Input: part model. Units: mm. Frame: model coordinates. A direction names the side the tool comes from. Round coordinates to 2 decimals unless told otherwise and drop trailing zeros. Loops run counter-clockwise (first coordinate to the right, second up) from the corner with the lowest first, then second, coordinate; pieces in that order, holes last. Notation, with made-up numbers: (26.5, 56.25) -> (37.5, 56.25) arc R19 ccw to (37.5, 67.25) -> close; hole circle Ø2 at (2, -22). An arc over 180 degrees is marked (long way). Answer in a Markdown table with one row per item. Add a question column.
Q1. Mould query, pull axis X, two halves, no side actions, for faces 1 (the face through (-6, -15, -6)), 2 (the face through (0.1, -4.4, 8.9)), 3 (the face through (-8.49, 3.69, -8.42)). Classes: pulls with the +X half, pulls with the -X half, needs draft (parallel to the pull), parting line crosses it, or undercut.
Q2. Section A-A, the plane y = 5. Output: boundary loops of the cut face in (x, z).
Q3. Section B-B, the plane y = -4. Output: boundary loops of the cut face in (x, z), and give its area (3 significant figures).
Q4. Reachability of faces 4 (the face through (-9, -11, -3.1)), 5 (the face through (6, -15, 6)), 6 (the face through (-6, -1, 6)), 7 (the face through (-3.8, -2.25, 0.04)) from +Z, -Z, +X, -X, +Y, -Y: full face, straight path, thin tool, end or side. Return the list, or none.
Q5. Pin query (flat end, axial travel): pin 1 (6 mm diameter, centred on y = 6, z = -5.5, fed in from +X); pin 2 (7.5 mm diameter, centred on y = -11, z = -10, fed in from -X); pin 3 (1.5 mm diameter, centred on x = -6.5, z = 5, fed in from +Y); pin 4 (3 mm diameter, centred on y = -10, z = -0.5, fed in from +X). Return the tip coordinate at first contact, or that it passes through.
Q6. Section C-C, the plane y = 9.5. Output: boundary loops of the cut face in (x, z), and give its area (3 significant figures).
Q7. Ray query, L1, parallel to Z at x = 7.5, y = -6.5; L2, parallel to Z at x = -6, y = 10; L3, parallel to X at y = -3.5, z = -3.25. Return the intervals inside material, ascending. Write a range as from..to.
Autodesk Inventor part; units mm, degrees
ref_plane "Work Plane2" through (0, 0, 0) normal (0.7071, 0, -0.7071) x (0, 1, 0)
ref_plane "XZ Plane" through (0, 0, 0) normal (0, 1, 0) x (-1, 0, 0)
sketch "Sketch1" plane through (0, 0, 0) normal (0, 1, 0) x (-1, 0, 0)
  circle A0 centre (0, 0) radius 12.5
  dimension "d0" = 25
extrude "Extrusion1" add sketch "Sketch1" along normal blind 19 and the other way blind 15
sketch "Sketch2" plane through (0, 0, 0) normal (0, 0, 1) x (1, 0, 0)
  line L0 (-5.25, -15) -> (-5.25, -7.5)
  arc A0 (5.25, -7.5) -> (-5.25, -7.5) centre (0, -7.5) ccw
  line L1 (5.25, -7.5) -> (5.25, -15)
  line L2 (5.25, -15) -> (-5.25, -15)
  line L3 (-3.1, -15) -> (-3.1, -7.5)
  arc A1 (3.1, -7.5) -> (-3.1, -7.5) centre (0, -7.5) ccw
  line L4 (3.1, -7.5) -> (3.1, -15)
  line L5 (0, 0) -> (0, -15) construction
  line L6 (-12.5, -15) -> (12.5, -15)
  point P0 (0, -7.5)
  dimension "d5" = 10.5
  dimension "d6" = 6.2
extrude "Extrusion2" cut sketch "Sketch2" along normal mid plane 10.5
extrude "Extrusion3" cut sketch "Sketch2" against normal through all both and the other way through all contours L3 A1 L4 L2
pattern_circular "Circular Pattern1" count 2 over 90 about axis through (0, -10, 0) along (0, 1, 0) of "Extrusion2", "Extrusion3"
ref_plane "Work Plane2" through (0, 0, 0) normal (0.7071, 0, -0.7071) x (0, 1, 0)
sketch "Sketch5" plane through (0, 0, 0) normal (0.7071, 0, -0.7071) x (0, 1, 0)
  line L0 (19, -21.9203) -> (-2.0622, -21.9203)
  line L1 (-21.8122, 0) -> (25.8729, 0)
  line L2 (19, -12.5) -> (19, 12.5)
  line L3 (19, -21.9203) -> (19, -4.9203)
  line L4 (19, -4.9203) -> (12, -4.9203)
  line L5 (12, -4.9203) -> (8.2472, -11.4203)
  line L6 (8.2472, -11.4203) -> (4, -11.4203)
  line L7 (4, -11.4203) -> (-2.0622, -21.9203)
  point P0 (0, 0)
  dimension "d40" = 21.9203
  dimension "d41" = 34
  dimension "d42" = 7
  dimension "d43" = 21
  dimension "d44" = 15
  dimension "d45" = 60
revolve "Revolution1" cut sketch "Sketch5" angle 360 about axis through (-15.5, 19, -15.5) along (0, -1, 0)
sketch "Sketch6" plane through (0, 19, 0) normal (0, 1, 0) x (1, 0, 0)
  circle A0 centre (6, 6) radius 1.9
  point P0 (0, 0)
  dimension "d47" = 3.8
  dimension "d48" = 6
  dimension "d49" = 6
extrude "Extrusion9" cut sketch "Sketch6" against normal blind 20
chamfer "Chamfer2" distance 0.5 angle 45 1 edges at (4.1, 19, -6)
pattern_circular "Circular Pattern4" count 2 over 360 about axis through (0, -10, 0) along (0, 1, 0) of "Revolution1", "Extrusion9", "Chamfer2"
chamfer "Chamfer1" distance 1 angle 45 4 edges at (8.8388, -15, 8.8388) (-8.8388, -15, 8.8388) (-8.8388, -15, -8.8388) (8.8388, -15, -8.8388)
properties part number "mount-stem_3DPrint"
Answer block:
| question | item | result |
|---|---|---|
| 1 | face 1 | needs draft |
| 1 | face 2 | undercut |
| 1 | face 3 | pulls with the -X half |
| 2 | outline | (-10.94, -6.04) arc R10.5 cw to (-6.04, -10.94) arc R12.5 ccw to (10.94, 6.04) arc R10.5 cw to (6.04, 10.94) arc R12.5 ccw to start; hole circle Ø3.8 at (-6, 6); hole circle Ø3.8 at (6, -6) |
| 3 | outline | circle Ø25 at (0, 0); hole (-5.25, -3.91) -> (-3.91, -3.91) -> (-3.91, -5.25) -> (3.91, -5.25) -> (3.91, -3.91) -> (5.25, -3.91) -> (5.25, 3.91) -> (3.91, 3.91) -> (3.91, 5.25) -> (-3.91, 5.25) -> (-3.91, 3.91) -> (-5.25, 3.91) -> close |
| 3 | area | 388 mm^2 |
| 4 | face 4 | +X, -X, -Y |
| 4 | face 5 | +Z, -Z, +X, -X, -Y |
| 4 | face 6 | +Y |
| 4 | face 7 | -Y |
| 5 | pin 1 | x = 12.25 |
| 5 | pin 2 | x = -10.83 |
| 5 | pin 3 | y = -1 |
| 5 | pin 4 | through |
| 6 | outline | (-12.05, -3.31) arc R12.67 cw to (-3.31, -12.05) arc R12.5 ccw to (12.05, 3.31) arc R12.67 cw to (3.31, 12.05) arc R12.5 ccw to start; hole circle Ø3.8 at (-6, 6); hole circle Ø3.8 at (6, -6) |
| 6 | area | 414 mm^2 |
| 7 | L1 | -10..-2.93, 2.93..10 |
| 7 | L2 | -5.86..4.1, 7.9..10.97 |
| 7 | L3 | -12.07..-5.25, 5.25..12.07 |
